from build123d import *

# Parameters (mm, degrees)
PAD009_DEPTH        = 8
HOLE001_D           = 5.5
HOLE001_DEPTH       = 25
HOLE001_CBORE_D     = 10
HOLE001_CBORE_DEPTH = 3
HOLE003_D           = 7.2
HOLE003_DEPTH       = 25
HOLE003_CBORE_D     = 12
HOLE003_CBORE_DEPTH = 3
SKETCH028_R         = 0.8
HOLE004_DEPTH       = 25
HOLE005_D           = 3.3
HOLE005_DEPTH       = 25
HOLE005_CBORE_D     = 6
HOLE005_CBORE_DEPTH = 1.8
SKETCH030_R         = 15
POCKET015_DEPTH     = 8.001
SKETCH031_R         = 0.8
HOLE006_DEPTH       = 25
SKETCH044_R         = 2.75
HOLE_DEPTH          = 25
SKETCH060_R         = 5
POCKET018_DEPTH     = 8.001
SKETCH061_R         = 0.8
HOLE023_DEPTH       = 25
SKETCH062_R         = 1.1
HOLE024_DEPTH       = 25


with BuildPart() as part:
    # Sketch023 (on Part) → Pad009 (new body)
    with BuildSketch(Plane.XY):
        with BuildLine():
            Line((-65.00001, 20.59), (65.00001, 20.59))
            ThreePointArc((70, 15.579804), (68.539147, 19.121927), (65.00001, 20.59))
            Line((70, 15.579804), (70, -124.420196))
            ThreePointArc((65.00001, -129.41), (68.531938, -127.949137), (70, -124.420196))
            Line((65.00001, -129.41), (-65.00001, -129.41))
            ThreePointArc((-70, -124.420196), (-68.531938, -127.949137), (-65.00001, -129.41))
            Line((-70, 15.579804), (-70, -124.420196))
            ThreePointArc((-65.00001, 20.59), (-68.539147, 19.121927), (-70, 15.579804))
        make_face()
    extrude(amount=PAD009_DEPTH)

    # Hole001
    with Locations(Plane.XY.offset(8)):
        with Locations((-48, -116.56), (48, -116.56)):
            CounterBoreHole(HOLE001_D / 2, HOLE001_CBORE_D / 2, HOLE001_CBORE_DEPTH, depth=HOLE001_DEPTH)

    # Hole003
    with Locations(Plane.XY.offset(8)):
        with Locations((-28, -56.56), (28, -56.56)):
            CounterBoreHole(HOLE003_D / 2, HOLE003_CBORE_D / 2, HOLE003_CBORE_DEPTH, depth=HOLE003_DEPTH)

    # Sketch028 (on Face5 of Hole003) → Hole004 (cut)
    with BuildSketch(Plane.XY.offset(8)):
        with Locations((-42, -35.56)):
            Circle(SKETCH028_R)
        with Locations((-14, -35.56)):
            Circle(SKETCH028_R)
        with Locations((14, -35.56)):
            Circle(SKETCH028_R)
        with Locations((42, -35.56)):
            Circle(SKETCH028_R)
        with Locations((-42, -50.56)):
            Circle(SKETCH028_R)
        with Locations((-14, -50.56)):
            Circle(SKETCH028_R)
        with Locations((14, -50.56)):
            Circle(SKETCH028_R)
        with Locations((42, -50.56)):
            Circle(SKETCH028_R)
        with Locations((-42, -65.56)):
            Circle(SKETCH028_R)
        with Locations((-14, -65.56)):
            Circle(SKETCH028_R)
        with Locations((14, -65.56)):
            Circle(SKETCH028_R)
        with Locations((42, -65.56)):
            Circle(SKETCH028_R)
        with Locations((-42, -80.56)):
            Circle(SKETCH028_R)
        with Locations((-14, -80.56)):
            Circle(SKETCH028_R)
        with Locations((14, -80.56)):
            Circle(SKETCH028_R)
        with Locations((42, -80.56)):
            Circle(SKETCH028_R)
        with Locations((-42, -95.56)):
            Circle(SKETCH028_R)
        with Locations((-14, -95.56)):
            Circle(SKETCH028_R)
        with Locations((14, -95.56)):
            Circle(SKETCH028_R)
        with Locations((42, -95.56)):
            Circle(SKETCH028_R)
    extrude(amount=-HOLE004_DEPTH, mode=Mode.SUBTRACT)

    # Hole005
    with Locations(Plane.XY.offset(8)):
        with Locations((-43.5, 6.59), (-12.5, 6.59), (-43.5, -24.41), (-12.5, -24.41), (12.5, 6.59), (43.5, 6.59), (12.5, -24.41), (43.5, -24.41)):
            CounterBoreHole(HOLE005_D / 2, HOLE005_CBORE_D / 2, HOLE005_CBORE_DEPTH, depth=HOLE005_DEPTH)

    # Sketch030 (on Face5 of Hole005) → Pocket015 (cut, through all)
    with BuildSketch(Plane.XY.offset(8)):
        with Locations((-28, -8.91)):
            Circle(SKETCH030_R)
        with Locations((28, -8.91)):
            Circle(SKETCH030_R)
    extrude(amount=-POCKET015_DEPTH, mode=Mode.SUBTRACT)

    # Sketch031 (on Face5 of Pocket015) → Hole006 (cut)
    with BuildSketch(Plane.XY.offset(8)):
        with Locations((-45.38, 16.99)):
            Circle(SKETCH031_R)
        with Locations((-38.62, 16.99)):
            Circle(SKETCH031_R)
        with Locations((-17.38, 16.99)):
            Circle(SKETCH031_R)
        with Locations((-10.62, 16.99)):
            Circle(SKETCH031_R)
        with Locations((10.62, 16.99)):
            Circle(SKETCH031_R)
        with Locations((17.38, 16.99)):
            Circle(SKETCH031_R)
        with Locations((38.62, 16.99)):
            Circle(SKETCH031_R)
        with Locations((45.38, 16.99)):
            Circle(SKETCH031_R)
    extrude(amount=-HOLE006_DEPTH, mode=Mode.SUBTRACT)

    # Sketch044 (on Face5 of Hole006) → Hole (cut)
    with BuildSketch(Plane.XY.offset(8)):
        with Locations((-65, -86.56)):
            Circle(SKETCH044_R)
        with Locations((65, -86.56)):
            Circle(SKETCH044_R)
    extrude(amount=-HOLE_DEPTH, mode=Mode.SUBTRACT)

    # Sketch060 → Pocket018 (cut, through all)
    with BuildSketch(Plane.XY):
        with Locations((-62, -34.420196)):
            Circle(SKETCH060_R)
        with Locations((62, -34.420196)):
            Circle(SKETCH060_R)
    extrude(amount=POCKET018_DEPTH, mode=Mode.SUBTRACT)

    # Sketch061 (on Face5 of Pocket018) → Hole023 (cut)
    with BuildSketch(Plane.XY.offset(8)):
        with Locations((-57, -66.56)):
            Circle(SKETCH061_R)
        with Locations((-57, -76.56)):
            Circle(SKETCH061_R)
        with Locations((57, -66.56)):
            Circle(SKETCH061_R)
        with Locations((57, -76.56)):
            Circle(SKETCH061_R)
    extrude(amount=-HOLE023_DEPTH, mode=Mode.SUBTRACT)

    # Sketch062 (on Face5 of Hole023) → Hole024 (cut)
    with BuildSketch(Plane.XY.offset(8)):
        with Locations((-65, -109.420196)):
            Circle(SKETCH062_R)
        with Locations((-65, -94.56)):
            Circle(SKETCH062_R)
        with Locations((65, -109.420196)):
            Circle(SKETCH062_R)
        with Locations((65, -94.56)):
            Circle(SKETCH062_R)
    extrude(amount=-HOLE024_DEPTH, mode=Mode.SUBTRACT)


solid = part.part
Can you work these out from the model? Positions are in its coordinate system, mm. A direction names the side the tool comes from. Round coordinates to 2 decimals unless told otherwise and drop trailing zeros. Write each loop counter-clockwise with the first axis right and the second up, starting at its lowest first coordinate (ties: lowest second). Pieces come first, ordered by that corner, then holes. Notation, with made-up numbers: (55.25, -9.75) -> (112.25, -9.75) arc R35 cw to (112.25, 26.25) -> close; hole circle Ø10 at (38, 0.25). An arc over 180 degrees is marked (long way). Use one line per item in the form item = value. Start each with the question number.
Q1. Imagine slicing it at A-A (y = -86.56). Please give me the cut outline in (x, z).
Q2. I'm going to push flat-ended pins straight in: P1, Ø1.4, axis at x = 14, y = -50.56, coming from the -Z side; P2, Ø3, axis at x = -12.5, y = 5.5, coming from the +Z side. Where does each tip first touch, or does it pass through?
Q3. Which directions (+Z, -Z, +X, -X, +Y, -Y) give clear straight access to the entire face, cutting with the end or side of a thin tool? Please do faces 1 (the face through (-11, -26, 6.2)), 2 (the face through (68.49, -127.99, 3.94)).
Q4. Imagine slicing it at C-C (z = 3.5). Count the separate pieces of the cut face and the enclosed holes in it, then the cut area to 3 significant figures.
Q5. If I drill on probe 1 along X at (y, z) = (-6.5, 1.5); probe 2 along Y at (x, z) = (-12.5, 4); probe 3 along Y at (x, z) = (-61.5, 2), over which ranges is the centre line in solid material (lowest first)? Write a range as [from, to].
Q6. Imagine slicing it at D-D (y = -4). Please give me the cut outline in (x, z).
Q7. Imagine slicing it at B-B (y = -116.56). Please give me the cut outline in (x, z).
Q8. We'd pull the mould along X, two halves only. Please class faces 3 (the face through (-70, -53, 4)), 4 (the face through (-42.985, -8.25, 4.056)), 5 (the face through (68.58, 19.08, 3.94)): +X half, -X half, draft (parallel to the pull), parting line (faces both ways), or undercut.
Worked out:
q1.outline = (-70, 0) -> (-67.75, 0) -> (-67.75, 8) -> (-70, 8) -> close; (-62.25, 0) -> (62.25, 0) -> (62.25, 8) -> (-62.25, 8) -> close; (67.75, 0) -> (70, 0) -> (70, 8) -> (67.75, 8) -> close
q2.P1 = through
q2.P2 = 6.2
q3.face_1 = +Z
q3.face_2 = +Z, -Z, +X, -Y
q4.separate_pieces = 1
q4.enclosed_holes = 54
q4.area = 19,100 mm^2
q5.probe_1 = [-70, -42.81], [-13.19, 13.19], [42.81, 70]
q5.probe_2 = [-129.41, -26.06], [-22.76, 4.94], [8.24, 20.59]
q5.probe_3 = [-129.41, -39.4], [-29.45, 20.59]
q6.outline = (-70, 0) -> (-42.17, 0) -> (-42.17, 8) -> (-70, 8) -> close; (-13.83, 0) -> (13.83, 0) -> (13.83, 8) -> (-13.83, 8) -> close; (42.17, 0) -> (70, 0) -> (70, 8) -> (42.17, 8) -> close
q7.outline = (-70, 0) -> (-50.75, 0) -> (-50.75, 5) -> (-53, 5) -> (-53, 8) -> (-70, 8) -> close; (-45.25, 0) -> (45.25, 0) -> (45.25, 5) -> (43, 5) -> (43, 8) -> (-43, 8) -> (-43, 5) -> (-45.25, 5) -> close; (50.75, 0) -> (70, 0) -> (70, 8) -> (53, 8) -> (53, 5) -> (50.75, 5) -> close
q8.face_3 = -X half
q8.face_4 = undercut
q8.face_5 = +X half
